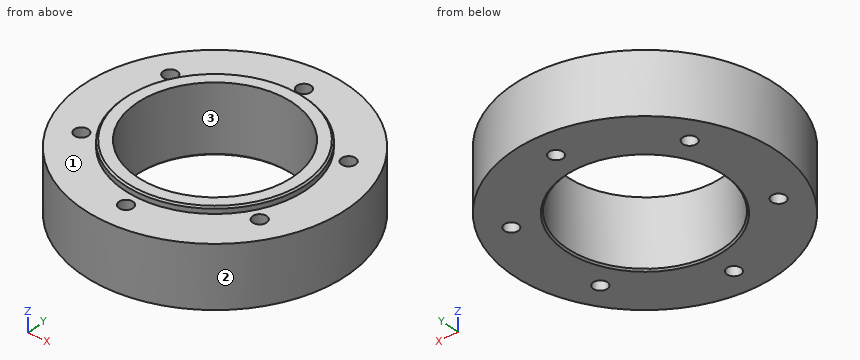
Autodesk Inventor part; units mm, degrees
ref_plane "YZ Plane" through (0, 0, 0) normal (1, 0, 0) x (0, 1, 0)
ref_plane "XZ Plane" through (0, 0, 0) normal (0, 1, 0) x (-1, 0, 0)
ref_plane "XY Plane" through (0, 0, 0) normal (0, 0, 1) x (1, 0, 0)
sketch "スケッチ1" plane through (0, 0, 0) normal (1, 0, 0) x (0, 1, 0)
  line L0 (40.5, 0) -> (24, 0)
  line L1 (24, 0) -> (24, -18.85)
  line L2 (24, -18.85) -> (40.5, -18.85)
  line L3 (40.5, -18.85) -> (40.5, 0)
  line L4 (0, -22.62) -> (0, 3.77)
  point P0 (0, 0)
  dimension "d0" = 24
  dimension "d2" = 40.5
  dimension "d3" = 18.85
revolve "回転1" add sketch "スケッチ1" angle 360 about axis through (0, 0, -10) along (0, 0, 1)
sketch "スケッチ2" plane through (0, 0, 0) normal (0, 0, 1) x (1, 0, 0)
  circle A0 centre (0, 0) radius 32
  point P0 (0, 32)
  point P1 (-27.7128, 16)
  point P2 (-27.7128, -16)
  point P3 (0, -32)
  point P4 (27.7128, -16)
  point P5 (27.7128, 16)
  dimension "d5" = 64
  dimension "d8" = 360
hole "穴1" at (0, 32, 0) at (-27.7128, 16, 0) at (-27.7128, -16, 0) at (0, -32, 0) at (27.7128, -16, 0) at (27.7128, 16, 0) direction (0, 0, -1) diameter 4.3 end through all
sketch "スケッチ5" plane through (0, 0, 0) normal (0, 0, 1) x (1, 0, 0)
  circle A0 centre (0, 0) radius 24
  circle A1 centre (0, 0) radius 28
  dimension "d28" = 4
extrude "押し出し3" add sketch "スケッチ5" along normal blind 2
chamfer "面取り1" distance 0.5 angle 45 1 edges at (-28, 0, 2)
chamfer "面取り2" distance 0.5 angle 45 1 edges at (0, -24, -18.85)
properties part number "unit-base7" material "ABS プラスチック"
Verification items for the finished model (mm, model axes). Face numbers are marked on the shaded views. Round coordinates to 2 decimals unless told otherwise and drop trailing zeros. Order: outer loops, then holes, each group sorted by start corner. A loop starts at its lowest first (then second) coordinate and runs counter-clockwise, first axis right, second up. Notation, with made-up numbers: (25.25, 59.25) - (61.25, 59.25) arc R17 cw to (61.25, 66.25) - close; hole circle Ø1 at (-26, 58.25). An arc over 180 degrees is marked (long way). Use CSV: the item, a comma, the result in double quotes.
(1) Mould release check, pull along Y, two halves, no side actions. Record for the marked faces 1, 2 and 3: released by +Y, released by -Y, zero draft, split by the parting line, or undercut.
Entries:
face 1,"zero draft"
face 2,"split by the parting line"
face 3,"undercut"
(2) Section check D-D on x = 32. Record the boundary of the cut face in (y, z).
Entries:
outline,"(-24.82, -18.85) - (24.82, -18.85) - (24.82, 0) - (-24.82, 0) - close"
(3) Section check A-A on y = 32. Record the boundary of the cut face in (x, z), and give its area (3 significant figures).
Entries:
outline,"(-24.82, -18.85) - (-2.15, -18.85) - (-2.15, 0) - (-24.82, 0) - close; (2.15, -18.85) - (24.82, -18.85) - (24.82, 0) - (2.15, 0) - close"
area,"855 mm^2"
(4) Section check B-B on z = -5.25. Record the boundary of the cut face in (x, y).
Entries:
outline,"circle Ø81 at (0, 0); hole circle Ø4.3 at (-27.71, -16); hole circle Ø4.3 at (-27.71, 16); hole circle Ø48 at (0, 0); hole circle Ø4.3 at (0, -32); hole circle Ø4.3 at (0, 32); hole circle Ø4.3 at (27.71, -16); hole circle Ø4.3 at (27.71, 16)"
(5) Section check C-C on y = -16. State how many separate pieces and enclosed holes the cut face has, and give its area (3 significant figures).
Entries:
separate pieces,"4"
enclosed holes,"0"
area,"586 mm^2"
(6) Gauge pin test, flat ends, axial feed: pin 1 Ø5 at (x, z) = (26.5, -3.5) entering from +Y; pin 2 Ø8 at (x, z) = (-17.5, -4) entering from -Y; pin 3 Ø7 at (x, y) = (27.71, 16) entering from +Z; pin 4 Ø3.5 at (x, y) = (-27.71, 16) entering from +Z. Record the tip position at first contact, or that the pin passes through.
Entries:
pin 1,"y = 32.62"
pin 2,"y = -38.18"
pin 3,"z = 0"
pin 4,"through"
(7) Thickness scan on probe 1 along Y at (x, z) = (0, -11.5); probe 2 along X at (y, z) = (16, -8); probe 3 along Z at (x, y) = (30, -26.5). Record the ranges inside material, lowest first. Write a range as from..to.
Entries:
probe 1,"-40.5..-34.15, -29.85..-24, 24..29.85, 34.15..40.5"
probe 2,"-37.21..-29.86, -25.56..-17.89, 17.89..25.56, 29.86..37.21"
probe 3,"-18.85..0"
